```python
from build123d import *

# Parameters (mm, degrees)
F0_W     = 200
F0_H     = 200
F1_DEPTH = 200
F2_R     = 40
F3_SCALE = 0.9


with BuildPart() as f1:
    # F0 (on Top) → F1 (new body)
    with BuildSketch(Plane.XY):
        Rectangle(F0_W, F0_H)
    extrude(amount=F1_DEPTH)

    # F2
    f2_edges = [f1.edges().sort_by_distance(p)[0] for p in [
        (-100, -100, 100),
        (100, -100, 100),
        (0, -100, 0),
        (0, -100, 200),
        (100, 100, 100),
        (-100, 100, 100),
        (0, 100, 0),
        (0, 100, 200),
        (100, 0, 0),
        (-100, 0, 0),
        (100, 0, 200),
        (-100, 0, 200),
    ]]
    fillet(f2_edges, radius=F2_R)


with BuildPart() as f3_1:
    # F3: copy of F1
    add(f1.part.scale(F3_SCALE))


with BuildPart() as f3_1_1:
    # F4: moved
    add(f3_1.part.moved(Location((0, 0, 10))))


with BuildPart() as f1_1:
    add(f1.part)

    # F5: cut F3_1
    add(f3_1_1.part, mode=Mode.SUBTRACT)


solid = f1_1.part
```
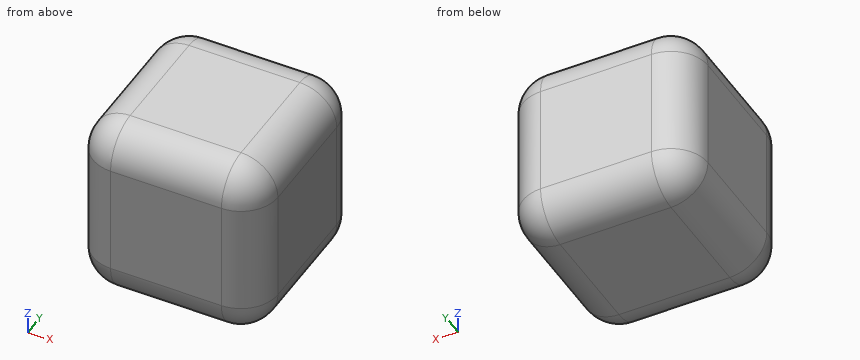
Geometry: final body of the model. Coordinates: model frame, mm. Give positions to 0.01 mm unless a question says otherwise; leave off trailing zeros. Loops run counter-clockwise (first coordinate to the right, second up) from the corner with the lowest first, then second, coordinate; pieces in that order, holes last. Notation, with made-up numbers: (-3, -33.75) -> (19, -33.75) arc R20 ccw to (19, -24.75) -> close; hole circle Ø2 at (-20, -25). An arc over 180 degrees is marked (long way). Return JSON: item names as keys, results as strings.
Item 1: Section A-A, the plane y = 27. Output: boundary loops of the cut face in (x, z), plus the area to 3 significant figures.
Filled in:
{"outline": "(-100, 40) arc R40 ccw to (-60, 0) -> (60, 0) arc R40 ccw to (100, 40) -> (100, 160) arc R40 ccw to (60, 200) -> (-60, 200) arc R40 ccw to (-100, 160) -> close; hole (-90, 46) arc R36 ccw to (-54, 10) -> (54, 10) arc R36 ccw to (90, 46) -> (90, 154) arc R36 ccw to (54, 190) -> (-54, 190) arc R36 ccw to (-90, 154) -> close", "area": "7,340 mm^2"}
Item 2: Pin query (flat end, axial travel): P1, Ø4, axis at x = 68.5, z = 130.5, coming from the +Y side; P2, Ø1.5, axis at x = 62, y = -64.5, coming from the -Z side; P3, Ø1.5, axis at y = -40, z = 38.5, coming from the +X side. Return the tip coordinate at first contact, or that it passes through.
Filled in:
{"P1": "y = 99.47", "P2": "z = 0.22", "P3": "x = 99.99"}
Item 3: Section B-B, the plane z = 113. Output: boundary loops of the cut face in (x, y).
Filled in:
{"outline": "(-100, -60) arc R40 ccw to (-60, -100) -> (60, -100) arc R40 ccw to (100, -60) -> (100, 60) arc R40 ccw to (60, 100) -> (-60, 100) arc R40 ccw to (-100, 60) -> close; hole (-90, -54) arc R36 ccw to (-54, -90) -> (54, -90) arc R36 ccw to (90, -54) -> (90, 54) arc R36 ccw to (54, 90) -> (-54, 90) arc R36 ccw to (-90, 54) -> close"}
Item 4: Line query: line 1 (Z direction, x = 18.5, y = 7); line 2 (Y direction, x = 25, z = 105). Output: solid intervals per line, ascending.
Filled in:
{"line 1": "0 to 10, 190 to 200", "line 2": "-100 to -90, 90 to 100"}
